Read the model definition and answer for the solid it produces. Units are mm, in the model's axes. Face numbers are marked on the shaded views. A direction names the side the tool comes from. Coordinates: 2 decimals unless noted, no trailing zeros. Order: outer loops, then holes, each group sorted by start corner. A loop starts at its lowest first (then second) coordinate and runs counter-clockwise, first axis right, second up. Notation, with made-up numbers: (-14.5, 42) -> (22.5, 42) arc R9 cw to (22.5, 52) -> close; hole circle Ø1 at (86, 35). An arc over 180 degrees is marked (long way). Return JSON: item names as keys, results as strings. Group by question number.
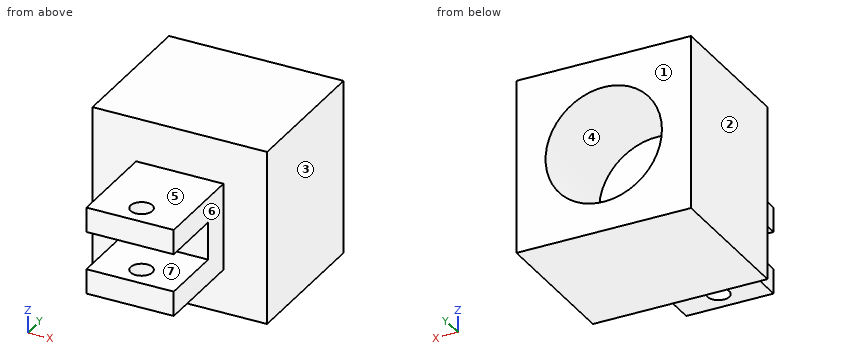
```python
from build123d import *

# Parameters (mm, degrees)
F0_W     = 6
F0_H     = 6.5
F0_R     = 0.75
F1_DEPTH = 3
F2_W     = 6
F2_H     = 6
F3_DEPTH = 1.3
F4_W     = 12
F4_H     = 12
F5_DEPTH = 10
F6_R     = 4
F7_DEPTH = 7


with BuildPart() as f1:
    # F0 (on Top) → F1 (new body, symmetric)
    with BuildSketch(Plane.XY):
        with Locations((0, 1.75)):
            Rectangle(F0_W, F0_H)
        Circle(F0_R, mode=Mode.SUBTRACT)
    extrude(amount=F1_DEPTH, both=True)

    # F2 (on Top) → F3 (cut, symmetric)
    with BuildSketch(Plane.XY):
        Rectangle(F2_W, F2_H)
    extrude(amount=F3_DEPTH, both=True, mode=Mode.SUBTRACT)

    # F4 (on face) → F5 (join)
    with BuildSketch(Plane(origin=(0, 5, 0), x_dir=(-1, 0, 0), z_dir=(0, 1, 0))):
        Rectangle(F4_W, F4_H)
    extrude(amount=F5_DEPTH)

    # F6 (on face) → F7 (cut)
    with BuildSketch(Plane(origin=(0, 15, 0), x_dir=(-1, 0, 0), z_dir=(0, 1, 0))):
        Circle(F6_R)
    extrude(amount=-F7_DEPTH, mode=Mode.SUBTRACT)


solid = f1.part
```
1. Find section C-C on z = 0. Determine the outline of the cut face in (x, y), and give its area (3 significant figures).
2. Which of the six approach directions +Z, -Z, +X, -X, +Y, -Y give full straight-line access (tool end or side, diameter ignored) to the marked faces 5, 6 and 7?
3. Find section B-B on x = 0. Determine the outline of the cut face in (y, z).
4. For a pull along X with two mould halves and no side action, classify the marked faces 1, 2, 3 and 4 as released by +X, released by -X, zero draft, split by the parting line, or undercut.
5. Find section D-D on y = 11. Determine the outline of the cut face in (x, z), and give its area (3 significant figures).
6. Find section A-A on y = 0. Determine the outline of the cut face in (x, z).
7. Given pin 1 (5 mm diameter, centred on x = 0, y = 0, fed in from -Z); pin 2 (4 mm diameter, centred on x = 2, z = -4, fed in from -Y); pin 3 (3 mm diameter, centred on x = -0.5, y = 0.5, fed in from +Z); pin 4 (2 mm diameter, centred on y = 1, z = 2, fed in from +X), each flat-ended and moving along its own axis, determine where each tip first touches the part or whether it passes through.
8. Straight lines are drawn through the part: L1, parallel to Z at x = 0, y = 11.75; L2, parallel to Y at x = 0, z = -1.6; L3, parallel to Y at x = -5.5, z = 0.25. For each, find the intervals that lie inside material, in ascending order.
Result:
{
 "1": {"outline": "(-6, 5) -> (-3, 5) -> (-3, 3) -> (3, 3) -> (3, 5) -> (6, 5) -> (6, 15) -> (4, 15) -> (4, 8) -> (-4, 8) -> (-4, 15) -> (-6, 15) -> close", "area": "76.0 mm^2"},
 "2": {"face 5": "+Z, +X, -X, -Y", "face 6": "+Z, -Z, +X, -Y", "face 7": "+X, -X, -Y"},
 "3": {"outline": "(-1.5, -3) -> (-0.75, -3) -> (-0.75, -1.3) -> (-1.5, -1.3) -> close; (-1.5, 1.3) -> (-0.75, 1.3) -> (-0.75, 3) -> (-1.5, 3) -> close; (0.75, -3) -> (5, -3) -> (5, -6) -> (15, -6) -> (15, -4) -> (8, -4) -> (8, 4) -> (15, 4) -> (15, 6) -> (5, 6) -> (5, 3) -> (0.75, 3) -> (0.75, 1.3) -> (3, 1.3) -> (3, -1.3) -> (0.75, -1.3) -> close"},
 "4": {"face 1": "zero draft", "face 2": "released by -X", "face 3": "released by +X", "face 4": "undercut"},
 "5": {"outline": "(-6, -6) -> (6, -6) -> (6, 6) -> (-6, 6) -> close; hole circle Ø8 at (0, 0)", "area": "93.7 mm^2"},
 "6": {"outline": "(-3, -3) -> (-0.75, -3) -> (-0.75, -1.3) -> (-3, -1.3) -> close; (-3, 1.3) -> (-0.75, 1.3) -> (-0.75, 3) -> (-3, 3) -> close; (0.75, -3) -> (3, -3) -> (3, -1.3) -> (0.75, -1.3) -> close; (0.75, 1.3) -> (3, 1.3) -> (3, 3) -> (0.75, 3) -> close"},
 "7": {"pin 1": "z = -3", "pin 2": "y = -1.5", "pin 3": "z = 3", "pin 4": "x = 3"},
 "8": {"L1": "-6 to -4, 4 to 6", "L2": "-1.5 to -0.75, 0.75 to 8", "L3": "5 to 15"}
}
